```python
from build123d import *

# Parameters (mm, degrees)
F0_R     = 12.7
F1_DEPTH = 25.4
F3_D     = 12.7
F4_R     = 1.27
F5_DEPTH = 12.701


with BuildPart() as f1:
    # F0 (on Top) → F1 (new body)
    with BuildSketch(Plane.XY):
        Circle(F0_R)
    extrude(amount=F1_DEPTH)

    # F3 (through all)
    with Locations(Plane.XY.offset(25.4)):
        with Locations((0, 0)):
            Hole(F3_D / 2)

    # F4 (on Front) → F5 (cut, through all)
    with BuildSketch(Plane.XZ):
        with Locations((0, 6.35)):
            Circle(F4_R)
        with Locations((0, 19.05)):
            Circle(F4_R)
    extrude(amount=F5_DEPTH, mode=Mode.SUBTRACT)


solid = f1.part
```
The listing builds one solid part. Answer for the finished solid, in the listing's coordinates (mm). A direction names the side the tool comes from. Give positions to 0.01 mm unless a question says otherwise; leave off trailing zeros. Order: outer loops, then holes, each group sorted by start corner. A loop starts at its lowest first (then second) coordinate and runs counter-clockwise, first axis right, second up. Notation, with made-up numbers: (54.5, -2) - (81.5, -2) arc R18 cw to (81.5, 21) - close; hole circle Ø9 at (60, 31). An arc over 180 degrees is marked (long way). Answer in a Markdown table with one row per item. Add a question column.
Q1. The part is cut by section D-D (z = 10). Determine the outline of the cut face in (x, y).
Q2. Given P1, Ø6, axis at y = 8, z = 12, coming from the -X side; P2, Ø6, axis at x = 7, z = 17, coming from the +Y side; P3, Ø1, axis at y = -4.5, z = 12, coming from the +X side, each flat-ended and moving along its own axis, determine where each tip first touches the part or whether it passes through.
Q3. For a pull along X with two mould halves and no side action, classify faces 3 (the cylindrical face through (-2.75, -12.4, 12.52)), 4 (the cylindrical face through (1.38, -6.2, 12.52)), 5 (the flat face through (3, 6, 25.4)) as released by +X, released by -X, zero draft, split by the parting line, or undercut.
Q4. Which of the six approach directions +Z, -Z, +X, -X, +Y, -Y give full straight-line access (tool end or side, diameter ignored) to faces 1 (the cylindrical face through (-0.17, -9.41, 20.31)), 2 (the flat face through (3, 6, 0))?
Q5. Find the intervals of material crossed by line 1 along Z through (x, y) = (0, -11.5); line 2 along Y through (x, z) = (0, 7.75); line 3 along Z through (x, y) = (-0.75, -9), in increasing order. Write a range as [from, to].
Q6. The part is cut by section C-C (x = 3). Determine the outline of the cut face in (y, z).
Q7. The part is cut by section B-B (x = 0). Determine the outline of the cut face in (y, z).
Q8. The part is cut by section A-A (y = 0). Determine the outline of the cut face in (x, z), then the cut area to 3 significant figures.
Determined:
| question | item | result |
|---|---|---|
| 1 | outline | circle Ø25.4 at (0, 0); hole circle Ø12.7 at (0, 0) |
| 2 | P1 | stops at x = -11.67 |
| 2 | P2 | stops at y = 12.05 |
| 2 | P3 | stops at x = 12.05 |
| 3 | face 3 | split by the parting line |
| 3 | face 4 | undercut |
| 3 | face 5 | zero draft |
| 4 | face 1 | -Y |
| 4 | face 2 | -Z, +X, -X, +Y, -Y |
| 5 | line 1 | z = [0, 5.08], [7.62, 17.78], [20.32, 25.4] |
| 5 | line 2 | y = [-12.7, -6.35], [6.35, 12.7] |
| 5 | line 3 | z = [0, 5.33], [7.37, 18.03], [20.07, 25.4] |
| 6 | outline | (-12.34, 0) - (-5.6, 0) - (-5.6, 25.4) - (-12.34, 25.4) - close; (5.6, 0) - (12.34, 0) - (12.34, 25.4) - (5.6, 25.4) - close |
| 7 | outline | (-12.7, 0) - (-6.35, 0) - (-6.35, 5.08) - (-12.7, 5.08) - close; (-12.7, 7.62) - (-6.35, 7.62) - (-6.35, 17.78) - (-12.7, 17.78) - close; (-12.7, 20.32) - (-6.35, 20.32) - (-6.35, 25.4) - (-12.7, 25.4) - close; (6.35, 0) - (12.7, 0) - (12.7, 25.4) - (6.35, 25.4) - close |
| 8 | outline | (-12.7, 0) - (-6.35, 0) - (-6.35, 25.4) - (-12.7, 25.4) - close; (6.35, 0) - (12.7, 0) - (12.7, 25.4) - (6.35, 25.4) - close |
| 8 | area | 323 mm² |
